from build123d import *

# Parameters (mm, degrees)
BASPROSKE_W                                       = 10
BASPROSKE_H                                       = 27
TOOTHCUT_DEPTH                                    = 40.471508712
TEETHCUTS_COUNT                                   = 25
TEETHCUTS_ANGLE                                   = 345.6
BORSKE_R                                          = 5
BORE_DEPTH                                        = 50.0000508
SKETCH2_R                                         = 15
BOSS_EXTRUDE1_DEPTH                               = 8
SKETCH3_R                                         = 6
CUT_EXTRUDE2_DEPTH                                = 8
CSK_FOR_M2_5_FLAT_HEAD_MACHINE_SCREW1_D           = 3.1
CSK_FOR_M2_5_FLAT_HEAD_MACHINE_SCREW1_DEPTH       = 18
CSK_FOR_M2_5_FLAT_HEAD_MACHINE_SCREW1_CSINK_D     = 5.5
CSK_FOR_M2_5_FLAT_HEAD_MACHINE_SCREW1_CSINK_ANGLE = 90
CSK_FOR_M2_5_FLAT_HEAD_MACHINE_SCREW1_TIP         = 0.931333959


with BuildPart() as part:
    # BasProSke → Base-Revolve (revolve)
    with BuildSketch(Plane(origin=(0, 0, 0), x_dir=(1, 0, 0), z_dir=(0, 1, 0)), mode=Mode.PRIVATE) as base_revolve_sk:
        with Locations((5, 13.5)):
            Rectangle(BASPROSKE_W, BASPROSKE_H)
    revolve(base_revolve_sk.sketch.rotate(Axis((-10, 0, 0), (1, 0, 0)), 180), axis=Axis((-10, 0, 0), (1, 0, 0)))

    # TooCutSke → ToothCut (cut, through all)
    with BuildSketch(Plane(origin=(0, 0, 0), x_dir=(0, 0, -1), z_dir=(1, 0, 0))):
        with BuildLine():
            ThreePointArc((0.946154762, 22.479096783), (0, 22.499), (-0.946154762, 22.479096783))
            ThreePointArc((-0.946154762, 22.479096783), (-1.62094792, 24.792268013), (-2.829470045, 26.876873784))
            ThreePointArc((-2.829470045, 26.876873784), (0, 27.0254), (2.829470045, 26.876873784))
            ThreePointArc((2.829470045, 26.876873784), (1.62094792, 24.792268013), (0.946154762, 22.479096783))
        make_face()
    toothcut = extrude(amount=TOOTHCUT_DEPTH, mode=Mode.SUBTRACT)

    # TeethCuts: ToothCut ×25 about axis
    teethcuts_axis = Axis((-10, 0, 0), (1, 0, 0))
    for i in range(1, TEETHCUTS_COUNT):
        add(toothcut.rotate(teethcuts_axis, i * TEETHCUTS_ANGLE / (TEETHCUTS_COUNT - 1)), mode=Mode.SUBTRACT)

    # BorSke → Bore (cut, symmetric)
    with BuildSketch(Plane(origin=(0, 0, 0), x_dir=(0, 0, -1), z_dir=(1, 0, 0))):
        with Locations(Location((0, 0, 0), (0, 0, 180))):
            Circle(BORSKE_R)
    extrude(amount=BORE_DEPTH, both=True, mode=Mode.SUBTRACT)

    # Sketch2 → Boss-Extrude1 (add)
    with BuildSketch(Plane.ZY):
        with Locations(Location((0, 0, 0), (0, 0, 180))):
            Circle(SKETCH2_R)
    extrude(amount=BOSS_EXTRUDE1_DEPTH)

    # Sketch3 → Cut-Extrude2 (cut)
    with BuildSketch(Plane.ZY.offset(8)):
        Circle(SKETCH3_R)
    extrude(amount=-CUT_EXTRUDE2_DEPTH, mode=Mode.SUBTRACT)

    # CSK for M2.5 Flat Head Machine Screw1
    with Locations(Plane.ZY.offset(8)):
        with Locations((12, 0), (8.485281374, -8.485281374), (0, -12), (-8.485281374, -8.485281374), (-12, 0), (-8.485281374, 8.485281374), (0, 12), (8.485281374, 8.485281374), (0, 0)):
            CounterSinkHole(CSK_FOR_M2_5_FLAT_HEAD_MACHINE_SCREW1_D / 2, CSK_FOR_M2_5_FLAT_HEAD_MACHINE_SCREW1_CSINK_D / 2, depth=CSK_FOR_M2_5_FLAT_HEAD_MACHINE_SCREW1_DEPTH, counter_sink_angle=CSK_FOR_M2_5_FLAT_HEAD_MACHINE_SCREW1_CSINK_ANGLE)
            with Locations((0, 0, -(CSK_FOR_M2_5_FLAT_HEAD_MACHINE_SCREW1_DEPTH + CSK_FOR_M2_5_FLAT_HEAD_MACHINE_SCREW1_TIP / 2))):  # 118° drill point
                Cone(0, CSK_FOR_M2_5_FLAT_HEAD_MACHINE_SCREW1_D / 2, CSK_FOR_M2_5_FLAT_HEAD_MACHINE_SCREW1_TIP, mode=Mode.SUBTRACT)


solid = part.part
Could you check a few things on this model? Use its own coordinates, in mm. A direction names the side the tool comes from. Coordinates: 2 decimals unless noted, no trailing zeros. Order: outer loops, then holes, each group sorted by start corner. A loop starts at its lowest first (then second) coordinate and runs counter-clockwise, first axis right, second up. Notation, with made-up numbers: (32, 77.5) - (80, 77.5) arc R28 ccw to (80, 97.5) - close; hole circle Ø10 at (-11.5, 64). An arc over 180 degrees is marked (long way). Answer in a Markdown table with one row per item. Add a question column.
(1) If we section it at A-A, the plane y = -12: Please give me the cut outline in (x, z).
(2) If we mould it in two halves opening along Z, with no side actions, what happens to faces 1 (the face through (4.93, 1.426, 22.454)), 2 (the face through (4.93, -14.35, -17.33))? For each: released by +Z, released by -Z, zero draft, split by the parting line, or undercut.
(3) If we section it at B-B, the plane x = -6: State how many separate pieces and enclosed holes the cut face has, then the cut area to 3 significant figures.
(4) On a 3-axis mill with a long thin cutter (end or side, diameter ignored), from which of +Z, -Z, +X, -X, +Y, -Y can I reach the whole of each face in a straight line? I mean faces 3 (the face through (4.93, -9.568, 20.363)), 4 (the face through (4.9, -24.8, -1.5)). Say none if no direction works.
(5) I need wall thicknesses on L1, parallel to Y at x = 3.75, z = 0; L2, parallel to Y at x = -4.25, z = -1; L3, parallel to X at y = -14.5, z = 11.5. Which ranges of each line are inside material? Lowest first, please.
(6) Will these pins go through, and if not, where does the flat tip stop? pin 1 (12 mm diameter, centred on y = -7, z = 20, fed in from -X); pin 2 (5 mm diameter, centred on x = -4, z = -12.5, fed in from -Y); pin 3 (3 mm diameter, centred on x = 6, z = -21.5, fed in from +Y).
Results are:
| question | item | result |
|---|---|---|
| 1 | outline | (-8, -9) - (0, -9) - (0, -21.72) - (10, -21.72) - (10, -1.55) - (-6.8, -1.55) - (-8, -2.75) - close; (-8, 2.75) - (-6.8, 1.55) - (10, 1.55) - (10, 21.72) - (0, 21.72) - (0, 9) - (-8, 9) - close |
| 2 | face 1 | released by +Z |
| 2 | face 2 | undercut |
| 3 | separate pieces | 1 |
| 3 | enclosed holes | 9 |
| 3 | area | 533 mm2 |
| 4 | face 3 | +X, -X |
| 4 | face 4 | +X, -X, -Y |
| 5 | L1 | y = -27 to -13.55, -10.45 to -5, 5 to 10.45, 13.55 to 22.5 |
| 5 | L2 | y = -14.97 to -13.18, -10.82 to -5.92, 5.92 to 10.82, 13.18 to 14.97 |
| 5 | L3 | x = 0 to 10 |
| 6 | pin 1 | stops at x = 0 |
| 6 | pin 2 | stops at y = -11.18 |
| 6 | pin 3 | stops at y = 17.65 |
